```python
from build123d import *

# Parameters (mm, degrees)
F0_R     = 19.25
F0_R_2   = 7
F1_DEPTH = 10


with BuildPart() as f1:
    # F0 (on Top) → F1 (new body)
    with BuildSketch(Plane.XY):
        Circle(F0_R)
        with BuildLine():
            ThreePointArc((7.896499, 9.689959), (11.290621, 5.363942), (12.5, 0))
            ThreePointArc((12.5, 0), (11.290621, -5.363942), (7.896499, -9.689959))
            ThreePointArc((7.896499, -9.689959), (8.159581, -10.230758), (8.25, -10.825318))
            ThreePointArc((8.25, -10.825318), (6.689887, -12.776343), (4.443501, -11.683548))
            ThreePointArc((4.443501, -11.683548), (0, -12.5), (-4.443501, -11.683548))
            ThreePointArc((-4.443501, -11.683548), (-7.25, -12.557368), (-7.896499, -9.689959))
            ThreePointArc((-7.896499, -9.689959), (-12.5, 0), (-7.896499, 9.689959))
            ThreePointArc((-7.896499, 9.689959), (-7.25, 12.557368), (-4.443501, 11.683548))
            ThreePointArc((-4.443501, 11.683548), (0, 12.5), (4.443501, 11.683548))
            ThreePointArc((4.443501, 11.683548), (6.689887, 12.776343), (8.25, 10.825318))
            ThreePointArc((8.25, 10.825318), (8.159581, 10.230758), (7.896499, 9.689959))
        make_face(mode=Mode.SUBTRACT)
        with BuildLine():
            ThreePointArc((7.896499, -9.689959), (11.290621, -5.363942), (12.5, 0))
            ThreePointArc((12.5, 0), (11.290621, 5.363942), (7.896499, 9.689959))
            ThreePointArc((7.896499, 9.689959), (5.25, 9.093267), (4.443501, 11.683548))
            ThreePointArc((4.443501, 11.683548), (0, 12.5), (-4.443501, 11.683548))
            ThreePointArc((-4.443501, 11.683548), (-4.298975, 11.265205), (-4.25, 10.825318))
            ThreePointArc((-4.25, 10.825318), (-5.655441, 8.915737), (-7.896499, 9.689959))
            ThreePointArc((-7.896499, 9.689959), (-12.5, 0), (-7.896499, -9.689959))
            ThreePointArc((-7.896499, -9.689959), (-5.655441, -8.915737), (-4.25, -10.825318))
            ThreePointArc((-4.25, -10.825318), (-4.298975, -11.265205), (-4.443501, -11.683548))
            ThreePointArc((-4.443501, -11.683548), (0, -12.5), (4.443501, -11.683548))
            ThreePointArc((4.443501, -11.683548), (5.25, -9.093267), (7.896499, -9.689959))
        make_face()
        Circle(F0_R_2, mode=Mode.SUBTRACT)
    extrude(amount=F1_DEPTH)


solid = f1.part
```
Verification items for the finished model (mm, model axes). Coordinates: 2 decimals unless noted, no trailing zeros. Order: outer loops, then holes, each group sorted by start corner. A loop starts at its lowest first (then second) coordinate and runs counter-clockwise, first axis right, second up. Notation, with made-up numbers: (-37.5, -29) -> (21.5, -29) arc R17 ccw to (21.5, 3) -> close; hole circle Ø10 at (13.5, 14.5). An arc over 180 degrees is marked (long way). Put each result on its own line as item: value. Start each with the question number.
1) Release check for a two-part mould opening along X. For faces 1 (the cylindrical face through (6.466, -2.681, 4.93)), 2 (the flat face through (0, -8, 10)), 3 (the cylindrical face through (-15.28, -11.71, 4.93)) record: pulls with the +X half, pulls with the -X half, needs draft (parallel to the pull), parting line crosses it, or undercut.
2) Cross-section at B-B (z = 5). Enter the section's corners in (x, y).
3) Cross-section at D-D (x = -6.25). Enter the section's corners in (y, z), plus the area to 3 significant figures.
4) Cross-section at A-A (y = 0). Enter the section's corners in (x, z).
5) Material ranges on L1, parallel to X at y = -11, z = 9.25; L2, parallel to Y at x = -5.5, z = 3.25; L3, parallel to Y at x = -7.5, z = 6.5, recorded low to high.
6) Go/stop test with flat-tipped pins: pin 1 (1.5 mm diameter, centred on y = 13, z = 8, fed in from +X); pin 2 (11 mm diameter, centred on x = 0, y = 0, fed in from -Z); pin 3 (2 mm diameter, centred on x = -2, z = 7.5, fed in from -Y). Record where each tip stops, or that it passes through.
Geometry check:
1. face 1: undercut
1. face 2: needs draft
1. face 3: parting line crosses it
2. outline: circle Ø38.5 at (0, 0); hole circle Ø14 at (0, 0); hole (-4.44, -11.68) arc R2 ccw to (-4.25, -10.83) arc R2 ccw (long way) to start; hole (-4.44, 11.68) arc R2 ccw (long way) to (-4.25, 10.83) arc R2 ccw to start; hole (7.9, -9.69) arc R2 ccw (long way) to (8.25, -10.83) arc R2 ccw to start; hole (7.9, 9.69) arc R2 ccw to (8.25, 10.83) arc R2 ccw (long way) to start
3. outline: (-18.21, 0) -> (-12.83, 0) -> (-12.83, 10) -> (-18.21, 10) -> close; (-8.83, 0) -> (-3.15, 0) -> (-3.15, 10) -> (-8.83, 10) -> close; (3.15, 0) -> (8.83, 0) -> (8.83, 10) -> (3.15, 10) -> close; (12.83, 0) -> (18.21, 0) -> (18.21, 10) -> (12.83, 10) -> close
3. area: 221 mm^2
4. outline: (-19.25, 0) -> (-7, 0) -> (-7, 10) -> (-19.25, 10) -> close; (7, 0) -> (19.25, 0) -> (19.25, 10) -> (7, 10) -> close
5. L1: x = -15.8 to -8.24, -4.26 to 4.26, 8.24 to 15.8
5. L2: y = -18.45 to -12.68, -8.97 to -4.33, 4.33 to 8.97, 12.68 to 18.45
5. L3: y = -17.73 to -12.39, -9.26 to 9.26, 12.39 to 17.73
6. pin 1: stops at x = 14.85
6. pin 2: passes through
6. pin 3: stops at y = -19.22
